Build history of the part. All positions in model axes, mm. A direction names the side the tool comes from. Round coordinates to 2 decimals unless told otherwise and drop trailing zeros. Write each loop counter-clockwise with the first axis right and the second up, starting at its lowest first coordinate (ties: lowest second). Pieces come first, ordered by that corner, then holes. Notation, with made-up numbers: (26.25, -33.75) - (32.25, -33.75) arc R23 ccw to (32.25, -23.75) - close; hole circle Ø7 at (17.25, 88). An arc over 180 degrees is marked (long way). One line per question, with ' | ' between items.
from build123d import *

# Parameters (mm, degrees)
ESQUISSE1_W             = 60
ESQUISSE1_H             = 105
BOSS_EXTRU_1_DEPTH      = 3
CONG_1_R                = 30
ESQUISSE2_R             = 15
ENL_V_MAT_EXTRU_1_DEPTH = 3
ESQUISSE3_W             = 2.740256741
ESQUISSE3_H             = 25
ENL_V_MAT_EXTRU_2_DEPTH = 3
CONG_2_R                = 30


with BuildPart() as part:
    # Esquisse1 → Boss.-Extru.1 (new body)
    with BuildSketch(Plane.XY):
        with Locations((30, 52.5)):
            Rectangle(ESQUISSE1_W, ESQUISSE1_H)
    extrude(amount=BOSS_EXTRU_1_DEPTH)

    # Congé1
    cong_1_edges = [part.edges().sort_by_distance(p)[0] for p in [
        (60, 0, 1.5),
        (0, 0, 1.5),
    ]]
    fillet(cong_1_edges, radius=CONG_1_R - 0.0001)  # a hair under: the kernel refuses the full size

    # Esquisse2 → Enlèv. mat.-Extru.1 (cut)
    with BuildSketch(Plane.XY.offset(3)):
        with Locations((30, 30)):
            Circle(ESQUISSE2_R)
    extrude(amount=-ENL_V_MAT_EXTRU_1_DEPTH, mode=Mode.SUBTRACT)

    # Esquisse3 → Enlèv. mat.-Extru.2 (cut)
    with BuildSketch(Plane.XY.offset(3)):
        with Locations((1.370128371, 42.5)):
            Rectangle(ESQUISSE3_W, ESQUISSE3_H)
        with Locations((1.370128371, 92.5)):
            Rectangle(ESQUISSE3_W, ESQUISSE3_H)
    extrude(amount=-ENL_V_MAT_EXTRU_2_DEPTH, mode=Mode.SUBTRACT)

    # Congé2
    cong_2_edges = [part.edges().sort_by_distance(p)[0] for p in [
        (60, 105, 1.5),
    ]]
    fillet(cong_2_edges, radius=CONG_2_R)


solid = part.part
Q1. Which spindle directions (+Z, -Z, +X, -X, +Y, -Y) get a long thin tool onto all of the face, cutting with end or side? Do faces 1 (the cylindrical face through (8.555, 9.021, 1.521)), 2 (the flat face through (1, 55, 2)), 3 (the flat face through (2.74, 92, 2)). Say none if no direction does.
Found:
face 1: +Z, -Z, -X, -Y | face 2: +Z, -Z, -X | face 3: +Z, -Z, -X, +Y
Q2. Saw through at D-D, the plane x = 7. List the corners of the cut face in (y, z).
Found:
outline: (10.74, 0) - (105, 0) - (105, 3) - (10.74, 3) - close
Q3. Saw through at B-B, the plane x = 32.5. List the corners of the cut face in (y, z), then the cut area to 3 significant figures.
Found:
outline: (0.1, 0) - (15.21, 0) - (15.21, 3) - (0.1, 3) - close; (44.79, 0) - (104.9, 0) - (104.9, 3) - (44.79, 3) - close | area: 226 mm^2
Q4. Saw through at C-C, the plane y = 53. List the corners of the cut face in (x, z), then the cut area to 3 significant figures.
Found:
outline: (2.74, 0) - (60, 0) - (60, 3) - (2.74, 3) - close | area: 172 mm^2
Q5. Drill centre lines: L1, parallel to Y at x = 20, z = 0.9; L2, parallel to X at y = 28, z = 2.5; L3, parallel to X at y = 37.5, z = 2.15. Where is each one in solid material? Low to high. Write a range as from..to.
Found:
L1: 1.72..18.82, 41.18..105 | L2: 0.07..15.13, 44.87..59.93 | L3: 2.74..17.01, 42.99..60
Q6. Drop flat-ended pins along their axis: pin 1 (1.4 mm diameter, centred on x = 1.5, z = 1.5, fed in from -Y); pin 2 (0.9 mm diameter, centred on y = 91, z = 2, fed in from -X); pin 3 (0.8 mm diameter, centred on x = 1, z = 1.5, fed in from +Y). Give the stop position or say it passes through.
Found:
pin 1: y = 18.72 | pin 2: x = 2.74 | pin 3: y = 80
